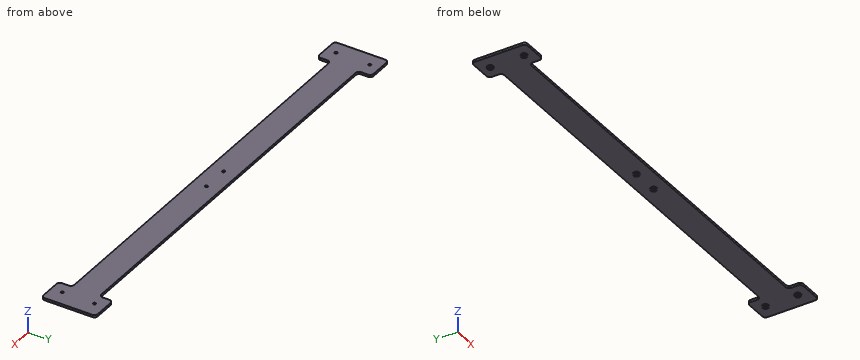
from build123d import *

# Parameters (mm, degrees)
F1_DEPTH = 3.42
F2_R     = 5
F3_R     = 4.5
F4_DEPTH = 5
F5_D     = 4.1


with BuildPart() as f1:
    # F0 (on Top) → F1 (new body)
    with BuildSketch(Plane.XY):
        Polygon((340.865, -40), (340.865, 40), (300.865, 40), (300.865, 20), (-300.865, 20), (-300.865, 40), (-340.865, 40), (-340.865, -40), (-300.865, -40), (-300.865, -20), (300.865, -20), (300.865, -40), align=None)
    extrude(amount=F1_DEPTH)

    # F2
    f2_edges = [f1.edges().sort_by_distance(p)[0] for p in [
        (-340.865, 40, 1.71),
        (-340.865, -40, 1.71),
        (-300.865, 40, 1.71),
        (-300.865, 20, 1.71),
        (-300.865, -20, 1.71),
        (-300.865, -40, 1.71),
        (300.865, 20, 1.71),
        (300.865, 40, 1.71),
        (340.865, 40, 1.71),
        (300.865, -40, 1.71),
        (300.865, -20, 1.71),
        (340.865, -40, 1.71),
    ]]
    fillet(f2_edges, radius=F2_R)

    # F3 (on face) → F4 (join)
    with BuildSketch(Plane.XY.offset(3.42)):
        with Locations((-320.865, 25)):
            Circle(F3_R)
        with Locations((-320.865, -25)):
            Circle(F3_R)
        with Locations((-20, 0)):
            Circle(F3_R)
        with Locations((20, 0)):
            Circle(F3_R)
        with Locations((318.0725574493, 23.9014066756)):
            Circle(F3_R)
        with Locations((318.0725574493, -23.9014066756)):
            Circle(F3_R)
    extrude(amount=-F4_DEPTH)

    # F5 (through all)
    with Locations(Plane.XY.offset(3.42)):
        with Locations((-320.865, -25), (-20, 0), (20, 0), (318.0725574493, 23.9014066756), (318.0725574493, -23.9014066756), (-320.865, 25)):
            Hole(F5_D / 2)


solid = f1.part
The listing builds one solid part. Answer for the finished solid, in the listing's coordinates (mm). Round coordinates to 2 decimals unless told otherwise and drop trailing zeros. Order: outer loops, then holes, each group sorted by start corner. A loop starts at its lowest first (then second) coordinate and runs counter-clockwise, first axis right, second up. Notation, with made-up numbers: (13.25, 3) -> (38.25, 3) arc R28 ccw to (38.25, 23) -> close; hole circle Ø5 at (26.5, 51.5). An arc over 180 degrees is marked (long way). Write each question's results on one line, items separated by ' | '. Start each with the question number.
Q1. Each of these flat-tipped pins is pushed along its axis until it touches: pin 1 (1 mm diameter, centred on x = -238.5, z = 1, fed in from -Y); pin 2 (6 mm diameter, centred on x = -272, y = 14.5, fed in from -Z); pin 3 (3.5 mm diameter, centred on x = -20, y = 0, fed in from +Z). Where does it stop, or does it pass through?
Q2. Straight lines are drawn through the part: probe 1 along X at (y, z) = (27.5, 0.2) (3 decimals); probe 2 along X at (y, z) = (23.5, 1.65) (3 decimals); probe 3 along Y at (x, z) = (-151, 2.4). For each, find the intervals that lie inside material, in ascending order. Write a range as from..to.
Q3. Find section A-A (z = 1.6). Give the number of separate pieces and of enclosed holes in the cut face, then the cut area to 3 significant figures.
Q4. Find section B-B (x = -211.5). Determine the outline of the cut face in (y, z).
Worked answers:
1) pin 1: stops at y = -20 | pin 2: stops at z = 0 | pin 3: passes through
2) probe 1: x = -340.865..-300.865, 300.865..340.865 | probe 2: x = -340.865..-322.262, -319.468..-300.635, 300.635..316.062, 320.083..340.865 | probe 3: y = -20..20
3) separate pieces: 1 | enclosed holes: 6 | area: 30,400 mm2
4) outline: (-20, 0) -> (20, 0) -> (20, 3.42) -> (-20, 3.42) -> close
